Autodesk Inventor part; units mm, degrees
ref_plane "YZ Plane" through (0, 0, 0) normal (1, 0, 0) x (0, 1, 0)
ref_plane "XZ Plane" through (0, 0, 0) normal (0, 1, 0) x (-1, 0, 0)
ref_plane "XY Plane" through (0, 0, 0) normal (0, 0, 1) x (1, 0, 0)
sketch "スケッチ1" plane through (0, 0, 0) normal (0, 0, 1) x (1, 0, 0)
  circle A0 centre (0, 0) radius 3.05
  circle A1 centre (0, 0) radius 11
  circle A2 centre (0, 0) radius 6.5
  circle A3 centre (0, 6.5) radius 2.5
  circle A4 centre (0, -6.5) radius 2.5
  circle A5 centre (6.5, 0) radius 2.5
  circle A6 centre (-6.5, 0) radius 2.5
  dimension "d0" = 6.1
  dimension "d1" = 22
  dimension "d2" = 13
  dimension "d3" = 5
  dimension "d4" = 5
  dimension "d5" = 5
  dimension "d6" = 5
extrude "押し出し1" add sketch "スケッチ1" along normal blind 5 contours A1 | A5 A2 A4 A6 A3
properties part number "passive_walking_robot6_parts2"
Geometry: final body of the model. Coordinates: model frame, mm. Give positions to 0.01 mm unless a question says otherwise; leave off trailing zeros. Order: outer loops, then holes, each group sorted by start corner. A loop starts at its lowest first (then second) coordinate and runs counter-clockwise, first axis right, second up. Notation, with made-up numbers: M -37.5,13.25 L 11.5,13.25 A9 cw 11.5,27.25 Z; hole C 43.25,83.25 d5. An arc over 180 degrees is marked long. Answer as CSV lines item,"result". Start each with the question number.
1) First-contact query: P1, Ø8, axis at x = 0, y = -6.5, coming from the +Z side; P2, Ø1, axis at x = -6, z = 4, coming from the +Y side; P3, Ø1, axis at x = 8.5, z = 4, coming from the -Y side; P4, Ø3, axis at x = 0, y = 6.5, coming from the +Z side. Flat tips, straight axial feed; report the tip coordinate or a pass-through.
2) Line query: line 1 (Y direction, x = 0, z = 2.1); line 2 (X direction, y = 2.25, z = 3.15); line 3 (X direction, y = -8.75, z = 1.15). Output: solid intervals per line, ascending. Write a range as from..to.
3) Mould query, pull axis X, two halves, no side actions, for faces 1 (the cylindrical face through (8.885, -0.751, 2.465)), 2 (the cylindrical face through (-2.38, 10.74, 2.46)), 3 (the flat face through (2.3, -2.3, 0)). Classes: +X half, -X half, draft (parallel to the pull), parting line (faces both ways), or undercut.
4) Cut plane A-A (x = 0). Output: boundary loops of the cut face in (y, z).
5) Cut plane D-D (x = 6.75). Output: boundary loops of the cut face in (y, z).
6) Cut plane C-C (y = 7.5). Output: boundary loops of the cut face in (x, z), then the cut area to 3 significant figures.
Findings below:
1,P1,"stops at z = 5"
1,P2,"stops at y = 9.53"
1,P3,"stops at y = -7.55"
1,P4,"passes through"
2,line 1,"y = -11..-9, -4..-3.05, 3.05..4, 9..11"
2,line 2,"x = -10.77..-7.59, -5.41..-2.06, 2.06..5.41, 7.59..10.77"
2,line 3,"x = -6.67..-1.09, 1.09..6.67"
3,face 1,"undercut"
3,face 2,"parting line"
3,face 3,"draft"
4,outline,"M -11,0 L -9,0 L -9,5 L -11,5 Z; M -4,0 L -3.05,0 L -3.05,5 L -4,5 Z; M 3.05,0 L 4,0 L 4,5 L 3.05,5 Z; M 9,0 L 11,0 L 11,5 L 9,5 Z"
5,outline,"M -8.69,0 L -2.49,0 L -2.49,5 L -8.69,5 Z; M 2.49,0 L 8.69,0 L 8.69,5 L 2.49,5 Z"
6,outline,"M -8.05,0 L -2.29,0 L -2.29,5 L -8.05,5 Z; M 2.29,0 L 8.05,0 L 8.05,5 L 2.29,5 Z"
6,area,"57.6 mm²"
